```python
from build123d import *

# Parameters (mm, degrees)
F0_W     = 42.7247285843
F0_H     = 49.0501485765
F1_DEPTH = 25
F2_R     = 5
F4_D     = 6.7564
F4_DEPTH = 9
F4_TIP   = 2.0298273432


with BuildPart() as f1:
    # F0 (on Front) → F1 (new body)
    with BuildSketch(Plane.XZ):
        with Locations((-69.0939426422, 50.483379513)):
            Rectangle(F0_W, F0_H)
    extrude(amount=F1_DEPTH)

    # F2
    f2_edges = [f1.edges().sort_by_distance(p)[0] for p in [
        (-47.731578, -12.5, 75.008454),
    ]]
    fillet(f2_edges, radius=F2_R)

    # F4
    with Locations(Plane.XZ.offset(25)):
        with Locations((-79.1495665908, 54.6661131084), (-60.4854077101, 47.1587516367)):
            Hole(F4_D / 2, depth=F4_DEPTH)
            with Locations((0, 0, -(F4_DEPTH + F4_TIP / 2))):  # 118° drill point
                Cone(0, F4_D / 2, F4_TIP, mode=Mode.SUBTRACT)


solid = f1.part
```
Read the model definition and answer for the solid it produces. Units are mm, in the model's axes. A direction names the side the tool comes from. Round coordinates to 2 decimals unless told otherwise and drop trailing zeros. Write each loop counter-clockwise with the first axis right and the second up, starting at its lowest first coordinate (ties: lowest second). Pieces come first, ordered by that corner, then holes. Notation, with made-up numbers: (29, 77.5) -> (45, 77.5) arc R34 ccw to (45, 114.5) -> close; hole circle Ø6 at (19.25, 65). An arc over 180 degrees is marked (long way). Answer in a Markdown table with one row per item. Add a question column.
1) Determine the mould class of faces 1 (the face through (-69, -12, 25.958)), 2 (the face through (-76.66, -20.44, 56.95)), 3 (the face through (-78.61, -14.32, 54.44)), 4 (the face through (-72, -12, 75.008)) for opening direction Z: pulls with the +Z half, pulls with the -Z half, needs draft (parallel to the pull), parting line crosses it, or undercut.
2) Consider line 1 (Z direction, x = -60, y = -22.75); line 2 (Z direction, x = -50, y = -16). Determine where each line is inside the solid, lowest interval first.
3) Find section A-A, the plane y = -23. Determine the outline of the cut face in (x, z).
4) Given P1, Ø1, axis at x = -59.5, z = 45, coming from the -Y side; P2, Ø4, axis at x = -60.49, z = 47.16, coming from the -Y side, each flat-ended and moving along its own axis, determine where each tip first touches the part or whether it passes through.
5) Which of the six approach directions +Z, -Z, +X, -X, +Y, -Y give full straight-line access (tool end or side, diameter ignored) to faces 5 (the face through (-63.606, -20.437, 45.865)), 6 (the face through (-90.456, -12, 50))?
Findings below:
| question | item | result |
|---|---|---|
| 1 | face 1 | pulls with the -Z half |
| 1 | face 2 | undercut |
| 1 | face 3 | undercut |
| 1 | face 4 | pulls with the +Z half |
| 2 | line 1 | 25.96 to 43.82, 50.5 to 75.01 |
| 2 | line 2 | 25.96 to 74.2 |
| 3 | outline | (-90.46, 25.96) -> (-47.73, 25.96) -> (-47.73, 70.01) arc R5 ccw to (-52.73, 75.01) -> (-90.46, 75.01) -> close; hole circle Ø6.76 at (-79.15, 54.67); hole circle Ø6.76 at (-60.49, 47.16) |
| 4 | P1 | y = -15.7 |
| 4 | P2 | y = -15.17 |
| 5 | face 5 | -Y |
| 5 | face 6 | +Z, -Z, -X, +Y, -Y |
